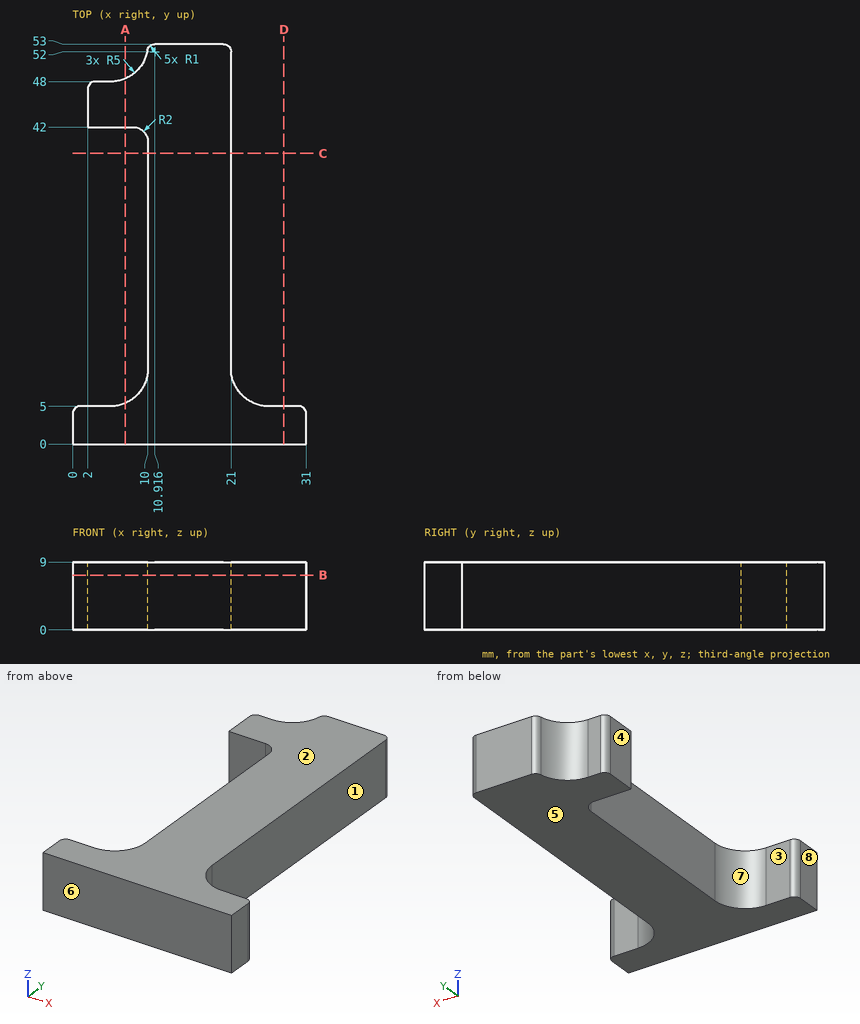
Design review of the part shown in the three views and the two pictorial views. Dimensions are in mm from the part's minimum x, y and z. A direction names the side the tool comes from. Coordinates: 2 decimals unless noted, no trailing zeros. Write each loop counter-clockwise with the first axis right and the second up, starting at its lowest first coordinate (ties: lowest second). Pieces come first, ordered by that corner, then holes.
(1) For pin 1 Ø3 at (x, z) = (6.5, 2) entering from -Y; pin 2 Ø2.5 at (y, z) = (23, 3.5) entering from +X; pin 3 Ø4 at (y, z) = (10, 4.5) entering from -X; pin 4 Ø1.2 at (x, z) = (28.5, 3.5) entering from +Y, all flat-tipped, find the tip position at first contact; note any pin that passes through.
(2) Add section B-B on z = 7.25. Give the boundary of the cut face in (x, y).
(3) Wall thickness on probe 1 along Y at (x, z) = (3.5, 7.25); probe 2 along X at (y, z) = (33, 6.25); probe 3 along Y at (x, z) = (29, 5.5): over which ranges is each line inside the solid? List them lowest first.
(4) The part is to be moulded in two halves that separate along Y. For the marked faces 6, 7 and 8, say which applies: +Y half, -Y half, draft (parallel to the pull), parting line (faces both ways), or undercut.
(5) Add section D-D on x = 28. Give the boundary of the cut face in (y, z).
(6) Add section A-A on x = 7. Give the boundary of the cut face in (y, z), then the cut area to 3 significant figures.
(7) Tool access review of the marked faces 1, 2, 3, 4 and 5: name each direction out of +Z, -Z, +X, -X, +Y, -Y from which nothing blocks a thin tool from reaching the whole face with its end or side.
(8) Add section C-C on y = 38.5. Give the boundary of the cut face in (x, z).
Answer sheet:
1. pin 1: stops at y = 0
1. pin 2: stops at x = 21
1. pin 3: stops at x = 9.58
1. pin 4: stops at y = 5
2. outline: (0, 0) - (31, 0) - (31, 4) arc R1 ccw to (30, 5) - (26, 5) arc R5 cw to (21, 10) - (21, 52) arc R1 ccw to (20, 53) - (10.92, 53) arc R1 ccw to (9.93, 52.17) arc R5 cw to (5, 48) - (3, 48) arc R1 ccw to (2, 47) - (2, 42) - (8, 42) arc R2 cw to (10, 40) - (10, 10) arc R5 cw to (5, 5) - (1, 5) arc R1 ccw to (0, 4) - close
3. probe 1: y = 0 to 5, 42 to 48
3. probe 2: x = 10 to 21
3. probe 3: y = 0 to 5
4. face 6: -Y half
4. face 7: undercut
4. face 8: draft
5. outline: (0, 0) - (5, 0) - (5, 9) - (0, 9) - close
6. outline: (0, 0) - (5.42, 0) - (5.42, 9) - (0, 9) - close; (42, 0) - (48.42, 0) - (48.42, 9) - (42, 9) - close
6. area: 107 mm2
7. face 1: +Z, -Z, +X, +Y
7. face 2: +Z, +X, -X, +Y, -Y
7. face 3: +Z, -Z, -X
7. face 4: +Z, -Z, -X, +Y
7. face 5: -Z, +X, -X, +Y, -Y
8. outline: (10, 0) - (21, 0) - (21, 9) - (10, 9) - close
